Check sheet for the modelled part. Datum: model origin and axes. Units: mm. Face numbers are marked on the shaded views. A direction names the side the tool comes from. Give positions to 0.01 mm unless a question says otherwise; leave off trailing zeros. Order: outer loops, then holes, each group sorted by start corner. A loop starts at its lowest first (then second) coordinate and runs counter-clockwise, first axis right, second up.
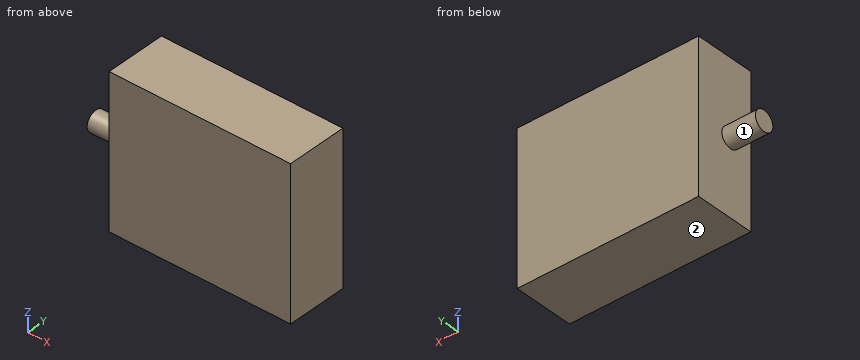
```python
from build123d import *

# Parameters (mm, degrees)
SKETCH1_W           = 27
SKETCH1_H           = 22.3
BOSS_EXTRUDE1_DEPTH = 9
SKETCH2_R           = 1.5
BOSS_EXTRUDE3_DEPTH = 5


with BuildPart() as part:
    # Sketch1 → Boss-Extrude1 (new body)
    with BuildSketch(Plane(origin=(0, 0, 0), x_dir=(1, 0, 0), z_dir=(0, 1, 0))):
        Rectangle(SKETCH1_W, SKETCH1_H)
    extrude(amount=BOSS_EXTRUDE1_DEPTH)

    # Sketch2 → Boss-Extrude3 (add)
    with BuildSketch(Plane.ZY.offset(13.5)):
        with Locations(Location((0, 3.5, 0), (0, 0, 180))):
            Circle(SKETCH2_R)
    extrude(amount=BOSS_EXTRUDE3_DEPTH)


solid = part.part
```
(1) Cross-section at D-D on z = 6.75. Enter the section's corners in (x, y), then the cut area to 3 significant figures.
Response values:
outline: (-13.5, 0) - (13.5, 0) - (13.5, 9) - (-13.5, 9) - close
area: 243 mm2
(2) Cross-section at B-B on z = 0. Enter the section's corners in (x, y), then the cut area to 3 significant figures.
Response values:
outline: (-18.5, 2) - (-13.5, 2) - (-13.5, 0) - (13.5, 0) - (13.5, 9) - (-13.5, 9) - (-13.5, 5) - (-18.5, 5) - close
area: 258 mm2
(3) Gauge pin test, flat end, axial feed: pin 1 Ø1 at (y, z) = (3, -3) entering from -X. Record the tip position at first contact, or that the pin passes through.
Response values:
pin 1: stops at x = -13.5
(4) Cross-section at C-C on y = 7. Enter the section's corners in (x, z).
Response values:
outline: (-13.5, -11.15) - (13.5, -11.15) - (13.5, 11.15) - (-13.5, 11.15) - close
(5) Material ranges on L1, parallel to X at y = 5.5, z = -1, recorded low to high.
Response values:
L1: x = -13.5 to 13.5
(6) Cross-section at A-A on y = 3.5. Enter the section's corners in (x, z), then the cut area to 3 significant figures.
Response values:
outline: (-18.5, -1.5) - (-13.5, -1.5) - (-13.5, -11.15) - (13.5, -11.15) - (13.5, 11.15) - (-13.5, 11.15) - (-13.5, 1.5) - (-18.5, 1.5) - close
area: 617 mm2
(7) Set-up check for the marked faces 1 and 2: record each of +Z, -Z, +X, -X, +Y, -Y from which the full face is reachable in a straight line by a thin tool's end or side.
Response values:
face 1: -X
face 2: -Z, +X, -X, +Y, -Y
